```python
from build123d import *

# Parameters (mm, degrees)
CUT_EXTRUDE1_DEPTH = 3.5
CHAMFER1_SIZE      = 0.5


with BuildPart() as part:
    # Sketch1 → Revolve1 (revolve)
    with BuildSketch(Plane.XY, mode=Mode.PRIVATE) as revolve1_sk:
        Polygon((0, 0), (29.5, 0), (29.5, 4), (4.5, 4), (1.5, 7), (0, 7), align=None)
    revolve(revolve1_sk.sketch.rotate(Axis((0, 0, 0), (1, 0, 0)), 90), axis=Axis((0, 0, 0), (1, 0, 0)))

    # Sketch2 → Cut-Extrude1 (cut)
    with BuildSketch(Plane.ZY):
        Polygon((0, 2.886751346), (-2.5, 1.443375673), (-2.5, -1.443375673), (0, -2.886751346), (2.5, -1.443375673), (2.5, 1.443375673), align=None)
    extrude(amount=-CUT_EXTRUDE1_DEPTH, mode=Mode.SUBTRACT)

    # Chamfer1
    chamfer1_edges = [part.edges().sort_by_distance(p)[0] for p in [
        (29.5, 0, -4),
    ]]
    chamfer(chamfer1_edges, length=CHAMFER1_SIZE)


solid = part.part
```
Part model, mm, in its own coordinate system. A direction names the side the tool comes from. Round coordinates to 2 decimals unless told otherwise and drop trailing zeros. Write each loop counter-clockwise with the first axis right and the second up, starting at its lowest first coordinate (ties: lowest second). Pieces come first, ordered by that corner, then holes.
Item 1: Two-plate mould, pull along Y, no slides. Class faces 1 (the flat face through (3.5, 0, 0)), 2 (the flat face through (0, 3.01, -0.1)), 3 (the conical face through (4.31, 3.72, 1.93)): +Y half, -Y half, draft (parallel to the pull), parting line (faces both ways), or undercut.
Results:
face 1: undercut
face 2: draft
face 3: parting line
Item 2: Probe L1, parallel to X at y = -2.25, z = 0.75; L2, parallel to X at y = 2, z = -5; L3, parallel to Y at x = 9, z = 0.75. List the from-to ranges inside material, lowest first.
Results:
L1: x = 3.5 to 29.5
L2: x = 0 to 3.11
L3: y = -3.93 to 3.93
Item 3: Cut at A-A, the plane x = 19.5. Give the cut face in (y, z).
Results:
outline: circle Ø8 at (0, 0)
Item 4: Which spindle directions (+Z, -Z, +X, -X, +Y, -Y) get a long thin tool onto all of the face, cutting with end or side? Do faces 4 (the cylindrical face through (0.74, 6.21, 3.23)), 5 (the flat face through (1.726, 2.175, -1.233)), 6 (the cylindrical face through (16.578, 3.905, -0.867)). Say none if no direction does.
Results:
face 4: +X, -X
face 5: -X
face 6: +X
Item 5: Drop flat-ended pins along their axis: pin 1 Ø0.9 at (x, y) = (2, 0.5) entering from +Z; pin 2 Ø5 at (x, y) = (18, 3.5) entering from +Z; pin 3 Ø4 at (x, y) = (13, 4.5) entering from -Z. Give the stop position or say it passes through.
Results:
pin 1: stops at z = 6.93
pin 2: stops at z = 3.87
pin 3: stops at z = -3.12
